The listing builds one solid part. Answer for the finished solid, in the listing's coordinates (mm). Face numbers are marked on the shaded views. Coordinates: 2 decimals unless noted, no trailing zeros. Order: outer loops, then holes, each group sorted by start corner. A loop starts at its lowest first (then second) coordinate and runs counter-clockwise, first axis right, second up. Notation, with made-up numbers: (7, -31) - (41, -31) arc R6 cw to (41, -24) - close; hole circle Ø2 at (38.5, -10). An arc over 180 degrees is marked (long way). One line per item, written item: value. Start each with the question number.
```python
from build123d import *

# Parameters (mm, degrees)
SKETCH1_W                                           = 38.1
SKETCH1_H                                           = 44.45
BOSS_EXTRUDE1_DEPTH                                 = 25.4
CSK_FOR_1_4_FLAT_HEAD_MACHINE_SCREW_100_D           = 6.7564
CSK_FOR_1_4_FLAT_HEAD_MACHINE_SCREW_100_CSINK_D     = 12.8778
CSK_FOR_1_4_FLAT_HEAD_MACHINE_SCREW_100_CSINK_ANGLE = 100
CSK_FOR_1_4_FLAT_HEAD_MACHINE_SCREW_2_D             = 6.7564
CSK_FOR_1_4_FLAT_HEAD_MACHINE_SCREW_2_CSINK_D       = 12.8778
CSK_FOR_1_4_FLAT_HEAD_MACHINE_SCREW_2_CSINK_ANGLE   = 100


# Read off the part's stored shape, not the designer's step: CSK for 1/4 Flat Head Machine Screw (100)3
with BuildPart() as part:
    # Sketch1 → Boss-Extrude1 (new body)
    with BuildSketch(Plane(origin=(0, 0, 0), x_dir=(1, 0, 0), z_dir=(0, 1, 0))):
        Rectangle(SKETCH1_W, SKETCH1_H)
    extrude(amount=BOSS_EXTRUDE1_DEPTH)

    # CSK for 1_4 Flat Head Machine Screw _100 (through all)
    with Locations(Plane(origin=(0, 25.4, 0), x_dir=(1, 0, 0), z_dir=(0, 1, 0))):
        with Locations((0, 9.525)):
            CounterSinkHole(CSK_FOR_1_4_FLAT_HEAD_MACHINE_SCREW_100_D / 2, CSK_FOR_1_4_FLAT_HEAD_MACHINE_SCREW_100_CSINK_D / 2, counter_sink_angle=CSK_FOR_1_4_FLAT_HEAD_MACHINE_SCREW_100_CSINK_ANGLE)

    # CSK for 1_4 Flat Head Machine Screw  2 (through all)
    with Locations(Plane.XZ):
        with Locations((0, 14.605)):
            CounterSinkHole(CSK_FOR_1_4_FLAT_HEAD_MACHINE_SCREW_2_D / 2, CSK_FOR_1_4_FLAT_HEAD_MACHINE_SCREW_2_CSINK_D / 2, counter_sink_angle=CSK_FOR_1_4_FLAT_HEAD_MACHINE_SCREW_2_CSINK_ANGLE)

    # CSK for 1_4 Flat Head Machine Screw 3 ou → CSK for 1_4 Flat Head Machine Screw  3 (revolve, cut)
    with BuildSketch(Plane(origin=(-11.43, 12.7, 0), x_dir=(1, 0, 0), z_dir=(0, -1, 0))):
        Polygon((0, -22.225), (3.3782, -22.225), (3.3782, 19.656767759), (6.4389, 22.225), (0, 22.225), align=None)
    revolve(axis=Axis((-11.43, 12.7, 0), (0, 0, 1)), mode=Mode.SUBTRACT)


solid = part.part
```
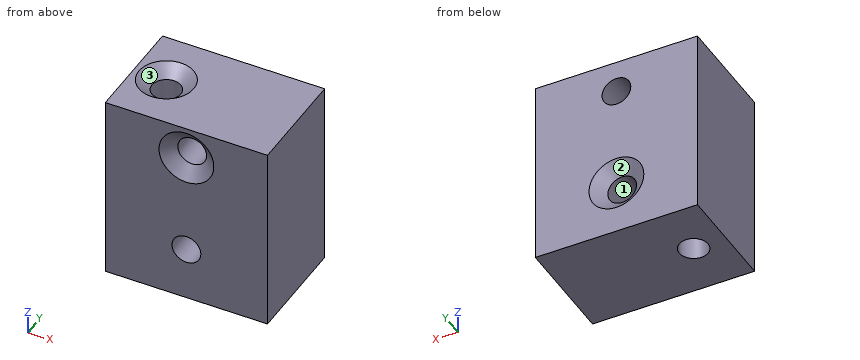
(1) The part is cut by section B-B on x = -11.43. Determine the outline of the cut face in (y, z) (3 decimals), plus the area to 3 significant figures.
(2) For a pull along Y with two mould halves and no side action, classify the marked faces 1, 2 and 3 as pulls with the +Y half, pulls with the -Y half, needs draft (parallel to the pull), parting line crosses it, or undercut.
(3) Flat-ended cylindrical pins translate along their axes: pin 1 Ø5.5 at (x, z) = (0, -9.525) entering from +Y; pin 2 Ø11 at (x, y) = (-11.43, 12.7) entering from +Z. Find the tip coordinate at first contact, or state that the pin passes through.
(4) Consider probe 1 along Z at (x, y) = (0, 13.25) (3 decimals); probe 2 along X at (y, z) = (14, 15.5); probe 3 along Y at (x, z) = (-11.43, 1.5). Determine where each line is inside the solid, lowest interval first.
(5) The part is cut by section A-A on x = 0. Determine the outline of the cut face in (y, z) (3 decimals), plus the area to 3 significant figures.
(6) The part is cut by section D-D on z = -2.5. Determine the outline of the cut face in (x, y).
(7) The part is cut by section C-C on y = 12.7. Determine the outline of the cut face in (x, z) (3 decimals).
Completed:
1. outline: (0, -22.225) - (9.322, -22.225) - (9.322, 19.657) - (6.261, 22.225) - (0, 22.225) - close; (16.078, -22.225) - (25.4, -22.225) - (25.4, 22.225) - (19.139, 22.225) - (16.078, 19.657) - close
1. area: 821 mm2
2. face 1: needs draft
2. face 2: pulls with the +Y half
2. face 3: undercut
3. pin 1: passes through
3. pin 2: stops at z = 21.44
4. probe 1: z = -22.225 to -12.903, -6.147 to 11.227, 17.983 to 22.225
4. probe 2: x = -19.05 to -14.55, -8.31 to -3.26, 3.26 to 19.05
4. probe 3: y = 0 to 9.32, 16.08 to 25.4
5. outline: (0, -22.225) - (25.4, -22.225) - (25.4, -15.964) - (22.832, -12.903) - (0, -12.903) - close; (0, -6.147) - (22.832, -6.147) - (25.4, -3.086) - (25.4, 11.227) - (2.568, 11.227) - (0, 8.166) - close; (0, 21.044) - (2.568, 17.983) - (25.4, 17.983) - (25.4, 22.225) - (0, 22.225) - close
5. area: 770 mm2
6. outline: (-19.05, 0) - (19.05, 0) - (19.05, 25.4) - (-19.05, 25.4) - close; hole circle Ø6.76 at (-11.43, 12.7)
7. outline: (-19.05, -22.225) - (-14.808, -22.225) - (-14.808, 19.657) - (-17.869, 22.225) - (-19.05, 22.225) - close; (-8.052, -22.225) - (19.05, -22.225) - (19.05, 22.225) - (-4.991, 22.225) - (-8.052, 19.657) - close; hole circle Ø6.756 at (0, -9.525); hole circle Ø6.756 at (0, 14.605)
